Check sheet for the drawn part. Datum: minimum x, y, z corner. Units: mm. A direction names the side the tool comes from. Give positions to 0.01 mm unless a question says otherwise; leave off trailing zeros. Order: outer loops, then holes, each group sorted by start corner. A loop starts at its lowest first (then second) coordinate and runs counter-clockwise, first axis right, second up.
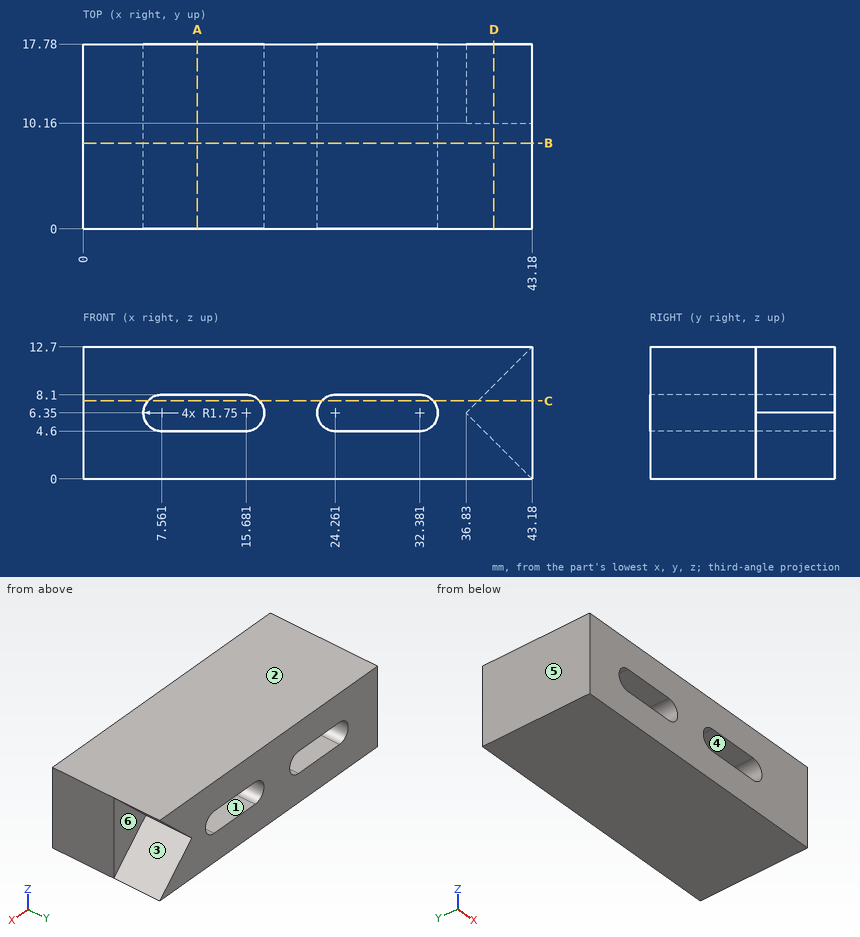
(1) Section check D-D, the plane x = 39.5. Enter the section's corners in (y, z).
Solved:
outline: (0, 0) - (17.78, 0) - (17.78, 3.68) - (10.16, 3.68) - (10.16, 9.02) - (17.78, 9.02) - (17.78, 12.7) - (0, 12.7) - close
(2) Section check B-B, the plane y = 8.25. Enter the section's corners in (x, z), then the cut area to 3 significant figures.
Solved:
outline: (0, 0) - (43.18, 0) - (43.18, 12.7) - (0, 12.7) - close; hole (7.56, 4.6) - (15.68, 4.6) arc R1.75 ccw to (15.68, 8.1) - (7.56, 8.1) arc R1.75 ccw to start; hole (24.26, 4.6) - (32.38, 4.6) arc R1.75 ccw to (32.38, 8.1) - (24.26, 8.1) arc R1.75 ccw to start
area: 472 mm2
(3) Release check for a two-part mould opening along X. For the marked faces 3, 4, 5 and 6 record: pulls with the +X half, pulls with the -X half, needs draft (parallel to the pull), parting line crosses it, or undercut.
Solved:
face 3: pulls with the +X half
face 4: undercut
face 5: pulls with the -X half
face 6: needs draft
(4) Go/stop test with a flat-tipped pin: pin 1 (1.9 mm diameter, centred on x = 41.5, z = 8.5, fed in from +Y). Record where the tip stops, or that it passes through.
Solved:
pin 1: stops at y = 10.16
(5) Set-up check for the marked faces 1 and 2: record each of +Z, -Z, +X, -X, +Y, -Y from which the full face is reachable in a straight line by a thin tool's end or side.
Solved:
face 1: +Y, -Y
face 2: +Z, +X, -X, +Y, -Y
(6) Section check C-C, the plane z = 7.5. Enter the section's corners in (x, y).
Solved:
outline: (0, 0) - (6.24, 0) - (6.24, 17.78) - (0, 17.78) - close; (17, 0) - (22.94, 0) - (22.94, 17.78) - (17, 17.78) - close; (33.7, 0) - (43.18, 0) - (43.18, 10.16) - (37.98, 10.16) - (37.98, 17.78) - (33.7, 17.78) - close
(7) Scan lines: line 1 (X direction, y = 7.25, z = 5.5); line 2 (Z direction, x = 10.5, y = 1); line 3 (X direction, y = 15.25, z = 6.25). Record each from-to range of solid material in increasing order.
Solved:
line 1: x = 0 to 6.03, 17.21 to 22.73, 33.91 to 43.18
line 2: z = 0 to 4.6, 8.1 to 12.7
line 3: x = 0 to 5.81, 17.43 to 22.51, 34.13 to 36.93
(8) Section check A-A, the plane x = 11. Enter the section's corners in (y, z).
Solved:
outline: (0, 0) - (17.78, 0) - (17.78, 4.6) - (0, 4.6) - close; (0, 8.1) - (17.78, 8.1) - (17.78, 12.7) - (0, 12.7) - close
